Can you work these out from the model? Positions are in its coordinate system, mm. A direction names the side the tool comes from. Give positions to 0.01 mm unless a question says otherwise; leave off trailing zeros. Write each loop counter-clockwise with the first axis right and the second up, starting at its lowest first coordinate (ties: lowest second). Pieces come first, ordered by that corner, then holes.
```python
from build123d import *

# Parameters (mm, degrees)
SKETCH1_W           = 52
SKETCH1_H           = 25
BOSS_EXTRUDE1_DEPTH = 29.75
CUT_EXTRUDE1_DEPTH  = 6
CUT_EXTRUDE2_REACH  = 43.44
SKETCH4_R           = 2.75
CUT_EXTRUDE3_REACH  = 45.841
SKETCH5_R           = 1.7
FILLET1_R           = 5
SKETCH6_R           = 3.5
CUT_EXTRUDE4_DEPTH  = 8


with BuildPart() as part:
    # Sketch1 → Boss-Extrude1 (new body)
    with BuildSketch(Plane(origin=(0, 0, 0), x_dir=(1, 0, 0), z_dir=(0, 1, 0))):
        Rectangle(SKETCH1_W, SKETCH1_H)
    extrude(amount=BOSS_EXTRUDE1_DEPTH)

    # Sketch2 → Cut-Extrude1 (cut)
    with BuildSketch(Plane.XY.offset(12.5)):
        with BuildLine():
            Line((19, 19.025), (6.525623627, 19.025))
            ThreePointArc((6.525623627, 19.025), (2.798843665, 19.593482447), (-0.588958859, 21.247222222))
            ThreePointArc((-0.588958859, 21.247222222), (-2.689396423, 22.272540883), (-5, 22.625))
            Line((-5, 22.625), (-12, 22.625))
            ThreePointArc((-12, 22.625), (-12.707106781, 22.332106781), (-13, 21.625))
            Line((-13, 21.625), (-13, 8.125))
            ThreePointArc((-13, 8.125), (-12.707106781, 7.417893219), (-12, 7.125))
            Line((-12, 7.125), (-5, 7.125))
            ThreePointArc((-5, 7.125), (-2.689396423, 7.477459117), (-0.588958859, 8.502777778))
            ThreePointArc((-0.588958859, 8.502777778), (2.798843665, 10.156517553), (6.525623627, 10.725))
            Line((6.525623627, 10.725), (19, 10.725))
            ThreePointArc((19, 10.725), (23.15, 14.875), (19, 19.025))
        make_face()
    extrude(amount=-CUT_EXTRUDE1_DEPTH, mode=Mode.SUBTRACT)

    # Sketch4 → Cut-Extrude2 (cut, up to next)
    with BuildSketch(Plane(origin=(0, 29.75, 0), x_dir=(1, 0, 0), z_dir=(0, 1, 0)), mode=Mode.PRIVATE) as cut_extrude2_sk1:
        with Locations(Location((-18, 1.5, 0), (0, 0, 270))):
            Circle(SKETCH4_R)
    cut_extrude2_tool1 = extrude(cut_extrude2_sk1.sketch, amount=-CUT_EXTRUDE2_REACH, mode=Mode.PRIVATE) & part.part
    # Sketch4 → Cut-Extrude2 (cut, up to next)
    with BuildSketch(Plane(origin=(0, 29.75, 0), x_dir=(1, 0, 0), z_dir=(0, 1, 0)), mode=Mode.PRIVATE) as cut_extrude2_sk2:
        with Locations(Location((7, 1.5, 0), (0, 0, 270))):
            Circle(SKETCH4_R)
    cut_extrude2_tool2 = extrude(cut_extrude2_sk2.sketch, amount=-CUT_EXTRUDE2_REACH, mode=Mode.PRIVATE) & part.part
    add(cut_extrude2_tool1.solids().sort_by_distance((-18, 29.75, -1.5))[0], mode=Mode.SUBTRACT)
    add(cut_extrude2_tool2.solids().sort_by_distance((7, 29.75, -1.5))[0], mode=Mode.SUBTRACT)

    # Sketch5 → Cut-Extrude3 (cut, up to next)
    with BuildSketch(Plane.XY.offset(6.5), mode=Mode.PRIVATE) as cut_extrude3_sk1:
        with Locations((-5, 14.875)):
            Circle(SKETCH5_R)
    cut_extrude3_tool1 = extrude(cut_extrude3_sk1.sketch, amount=-CUT_EXTRUDE3_REACH, mode=Mode.PRIVATE) & part.part
    # Sketch5 → Cut-Extrude3 (cut, up to next)
    with BuildSketch(Plane.XY.offset(6.5), mode=Mode.PRIVATE) as cut_extrude3_sk2:
        with Locations((19, 14.875)):
            Circle(SKETCH5_R)
    cut_extrude3_tool2 = extrude(cut_extrude3_sk2.sketch, amount=-CUT_EXTRUDE3_REACH, mode=Mode.PRIVATE) & part.part
    add(cut_extrude3_tool1.solids().sort_by_distance((-5, 14.875, 6.5))[0], mode=Mode.SUBTRACT)
    add(cut_extrude3_tool2.solids().sort_by_distance((19, 14.875, 6.5))[0], mode=Mode.SUBTRACT)

    # Fillet1
    fillet1_edges = [part.edges().sort_by_distance(p)[0] for p in [
        (-26, 14.875, 12.5),
        (-26, 14.875, -12.5),
    ]]
    fillet(fillet1_edges, radius=FILLET1_R)

    # Sketch6 → Cut-Extrude4 (cut)
    with BuildSketch(Plane(origin=(0, 0, -12.5), x_dir=(-1, 0, 0), z_dir=(0, 0, -1))):
        with Locations((-19, 14.875)):
            Circle(SKETCH6_R)
        with Locations((5, 14.875)):
            Circle(SKETCH6_R)
    extrude(amount=-CUT_EXTRUDE4_DEPTH, mode=Mode.SUBTRACT)


solid = part.part
```
1) Suppose I cut it at B-B on z = 10.5. Write out the boundary of the cut face in (x, y) (3 decimals).
Values follow:
outline: (-25, 0) - (26, 0) - (26, 29.75) - (-25, 29.75) - close; hole (-13, 8.125) arc R1 ccw to (-12, 7.125) - (-5, 7.125) arc R7.75 ccw to (-0.589, 8.503) arc R12.5 cw to (6.526, 10.725) - (19, 10.725) arc R4.15 ccw to (19, 19.025) - (6.526, 19.025) arc R12.5 cw to (-0.589, 21.247) arc R7.75 ccw to (-5, 22.625) - (-12, 22.625) arc R1 ccw to (-13, 21.625) - close
2) Suppose I cut it at D-D on z = -0.5. Write out the boundary of the cut face in (x, y) (3 decimals), plus the area to 3 significant figures.
Values follow:
outline: (-26, 0) - (-20.562, 0) - (-20.562, 29.75) - (-26, 29.75) - close; (-15.438, 0) - (4.438, 0) - (4.438, 29.75) - (-15.438, 29.75) - close; (9.562, 0) - (26, 0) - (26, 29.75) - (9.562, 29.75) - close; hole circle Ø3.4 at (-5, 14.875); hole circle Ø3.4 at (19, 14.875)
area: 1,220 mm2
3) Suppose I cut it at A-A on x = -18. Write out the boundary of the cut face in (y, z).
Values follow:
outline: (0, -12.5) - (29.75, -12.5) - (29.75, -4.25) - (0, -4.25) - close; (0, 1.25) - (29.75, 1.25) - (29.75, 12.5) - (0, 12.5) - close
4) For pin 1 Ø8 at (x, y) = (19, 14.875) entering from +Z; pin 2 Ø5 at (x, z) = (-18, -1.5) entering from +Y; pin 3 Ø6.5 at (x, z) = (7, -1.5) entering from -Y; pin 4 Ø2 at (x, y) = (20, 16) entering from -Z, each with a flat end and sliding along its axis, tell me the tip position at first contact or that it passes through.
Values follow:
pin 1: stops at z = 6.5
pin 2: passes through
pin 3: stops at y = 0
pin 4: stops at z = -4.5
5) If we mould it in two halves opening along Z, with no side actions, what happens to faces 1 (the face through (-24.57, 15.08, -11)), 2 (the face through (-15.273, 15.083, -1.858)), 3 (the face through (-5.369, 13.215, 1.077)), 4 (the face through (9.32, 15.08, -0.02))? For each: +Z half, -Z half, draft (parallel to the pull), parting line (faces both ways), or undercut.
Values follow:
face 1: -Z half
face 2: undercut
face 3: draft
face 4: undercut
6) Please list where these lines run through material, in increasing order: L1, parallel to X at y = 27, z = -1.75; L2, parallel to X at y = 11.5, z = -2.5; L3, parallel to X at y = 6.5, z = -7.75.
Values follow:
L1: x = -26 to -20.74, -15.26 to 4.26, 9.74 to 26
L2: x = -26 to -20.56, -15.44 to 4.44, 9.56 to 26
L3: x = -25.99 to 26
7) Suppose I cut it at C-C on y = 26.5. Write out the boundary of the cut face in (x, z).
Values follow:
outline: (-26, -7.5) arc R5 ccw to (-21, -12.5) - (26, -12.5) - (26, 12.5) - (-21, 12.5) arc R5 ccw to (-26, 7.5) - close; hole circle Ø5.5 at (-18, -1.5); hole circle Ø5.5 at (7, -1.5)
8) For faces 5 (the face through (-8.23, 13.53, -8.56)), 6 (the face through (-12.715, 7.426, 9.542)), 7 (the face through (-24.57, 15.08, 11)), which set-ups out of +Z, -Z, +X, -X, +Y, -Y let a thin tool reach every point of the face, with its end or its side?
Values follow:
face 5: -Z
face 6: +Z
face 7: +Z, -X, +Y, -Y
